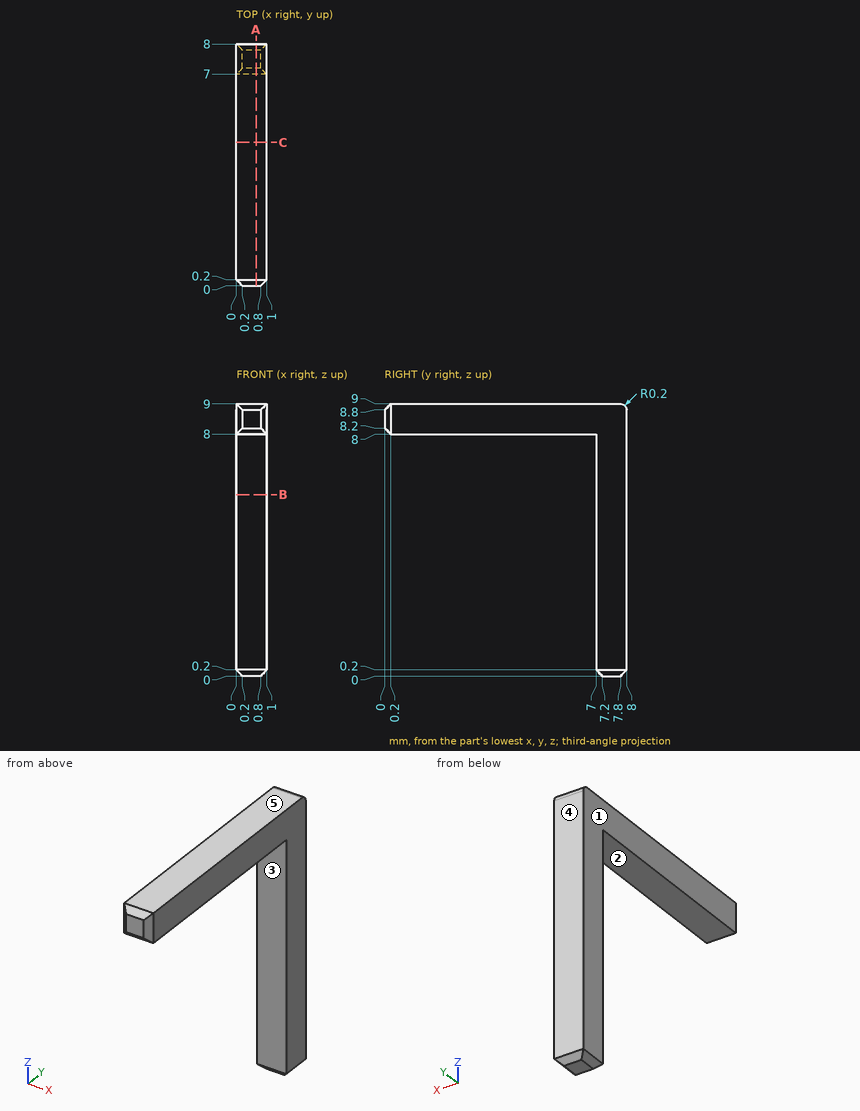
Geometry check sheet. Reference: drawing and pictorial views, mm from the part's lowest x, y, z. A direction names the side the tool comes from. Give positions to 0.01 mm unless a question says otherwise; leave off trailing zeros. Order: outer loops, then holes, each group sorted by start corner. A loop starts at its lowest first (then second) coordinate and runs counter-clockwise, first axis right, second up. Notation, with made-up numbers: M -17,23 L -7,23 A15 cw -7,49 Z; hole C -15,82 d5. An arc over 180 degrees is marked long. Use one line per item in the form item = value. Start each with the question number.
Q1. Scan lines: line 1 along Z through (x, y) = (0.75, 5); line 2 along Y through (x, z) = (0.4, 6.75). Record each from-to range of solid material in increasing order. Write a range as [from, to].
Q2. Section check C-C (y = 4.75). Enter the section's corners in (x, z), then the cut area to 3 significant figures.
Q3. Mould release check, pull along Y, two halves, no side actions. Record for the marked faces 3, 4 and 5: +Y half, -Y half, draft (parallel to the pull), parting line (faces both ways), or undercut.
Q4. Section check B-B (z = 6). Enter the section's corners in (x, y).
Q5. Section check A-A (x = 0.65). Enter the section's corners in (y, z).
Q6. Access from +Z, -Z, +X, -X, +Y, -Y to the whole of each face (thin tool, end or side, straight path). Record for the marked faces 1 and 2.
Evaluation:
q1.line_1 = [8, 9]
q1.line_2 = [7, 8]
q2.outline = M 0,8 L 1,8 L 1,9 L 0,9 Z
q2.area = 1.00 mm2
q3.face_3 = -Y half
q3.face_4 = +Y half
q3.face_5 = draft
q4.outline = M 0,7 L 1,7 L 1,8 L 0,8 Z
q5.outline = M 0,8.2 L 0.2,8 L 7,8 L 7,0.2 L 7.2,0 L 7.8,0 L 8,0.2 L 8,8.8 A0.2 ccw 7.8,9 L 0.2,9 L 0,8.8 Z
q6.face_1 = +Z, -Z, -X, +Y, -Y
q6.face_2 = -Z, +X, -X, -Y
